Verification items for the finished model (mm, model axes). A direction names the side the tool comes from. Coordinates: 2 decimals unless noted, no trailing zeros. Order: outer loops, then holes, each group sorted by start corner. A loop starts at its lowest first (then second) coordinate and runs counter-clockwise, first axis right, second up. Notation, with made-up numbers: M 2,-2 L 43,-2 A18 cw 43,21 Z; hole C 68.25,-11.75 d6. An arc over 180 degrees is marked long. Return JSON: item names as keys, results as strings. Group by question number.
1. Section check D-D, the plane y = 8.5. Record the cut outline in (x, z).
2. Section check A-A, the plane z = 70. Record the cut outline in (x, y).
3. Material ranges on line 1 along X through (y, z) = (36, 40.5); line 2 along Z through (x, y) = (41.5, 30); line 3 along Y through (x, z) = (-38, 90), recorded low to high.
4. Gauge pin test, flat ends, axial feed: pin 1 (10 mm diameter, centred on x = -9.5, y = 20, fed in from -Z); pin 2 (22 mm diameter, centred on y = 31, z = 50.5, fed in from +X); pin 3 (7 mm diameter, centred on y = 37, z = 79.5, fed in from -X). Record the tip position at first contact, or that the pin passes through.
5. Section check B-B, the plane x = 20. Record the cut outline in (y, z).
6. Set-up check for faces 1 (the cylindrical face through (40.56, 20.917, -6.377)), 2 (the flat face through (-14, 25.981, 15)), 3 (the flat face through (-40, 33, 69)): record each of +Z, -Z, +X, -X, +Y, -Y from which the full face is reachable in a straight line by a thin tool's end or side.
7. Section check C-C, the plane z = 50. Record the cut outline in (x, y), plus the area to 3 significant figures.
8. Mould release check, pull along X, two halves, no side actions. Record for faces 4 (the cylindrical face through (-29.191, -19.984, 69.44)), 5 (the cylindrical face through (56.315, 36.292, -7.465)), 6 (the flat face through (80, 19, -11)), 7 (the flat face through (41, 34, 10)): +X half, -X half, draft (parallel to the pull), parting line (faces both ways), or undercut.
```python
from build123d import *

# Parameters (mm, degrees)
BOSS_EXTRUDE1_DEPTH = 80
SKETCH2_R           = 5
CUT_EXTRUDE1_DEPTH  = 10
FILLET2_R           = 5
FILLET3_R           = 10
BOSS_EXTRUDE2_START = 25.98076
BOSS_EXTRUDE2_DEPTH = 16.932117
FILLET4_R           = 20
FILLET5_R           = 25
SKETCH6_W           = 5
SKETCH6_H           = 16.932118475
BOSS_EXTRUDE4_DEPTH = 80
SKETCH7_R           = 5
CUT_EXTRUDE2_DEPTH  = 40


with BuildPart() as part:
    # Sketch1 → Boss-Extrude1 (new body)
    with BuildSketch(Plane(origin=(0, 0, 0), x_dir=(0, 0, -1), z_dir=(1, 0, 0))):
        with BuildLine():
            Line((-10, 22.912878475), (-10, 42.912878475))
            Line((-10, 42.912878475), (-5, 42.912878475))
            Line((-5, 42.912878475), (-5, 19.364916731))
            ThreePointArc((-5, 19.364916731), (0, -20), (5, 19.364916731))
            Line((5, 19.364916731), (5, 42.912878475))
            Line((5, 42.912878475), (10, 42.912878475))
            Line((10, 42.912878475), (10, 22.912878475))
            ThreePointArc((10, 22.912878475), (0, -25), (-10, 22.912878475))
        make_face()
    extrude(amount=BOSS_EXTRUDE1_DEPTH)

    # Sketch2 → Cut-Extrude1 (cut, symmetric)
    with BuildSketch(Plane.XY):
        with Locations((20, 32.912878475)):
            Circle(SKETCH2_R)
        with Locations((60, 32.912878475)):
            Circle(SKETCH2_R)
    extrude(amount=CUT_EXTRUDE1_DEPTH, both=True, mode=Mode.SUBTRACT)

    # Fillet2
    fillet2_edges = [part.edges().sort_by_distance(p)[0] for p in [
        (40, 22.912878475, -10),
        (40, 22.912878475, 10),
    ]]
    fillet(fillet2_edges, radius=FILLET2_R)

    # Fillet3
    fillet3_edges = [part.edges().sort_by_distance(p)[0] for p in [
        (40, 19.364916731, 5),
        (40, 19.364916731, -5),
    ]]
    fillet(fillet3_edges, radius=FILLET3_R)

    # Sketch3 → Boss-Extrude2 (add)
    with BuildSketch(Plane(origin=(0, 0, 0), x_dir=(1, 0, 0), z_dir=(0, 1, 0)).offset(BOSS_EXTRUDE2_START)):
        Polygon((0, -10), (-20, -10), (-20, -30), (-25, -30), (-25, -5), (0, -5), align=None)
    extrude(amount=BOSS_EXTRUDE2_DEPTH)

    # Fillet4
    fillet4_edges = [part.edges().sort_by_distance(p)[0] for p in [
        (-20, 34.4468185, 10),
    ]]
    fillet(fillet4_edges, radius=FILLET4_R - 0.0001)  # a hair under: the kernel refuses the full size

    # Fillet5
    fillet5_edges = [part.edges().sort_by_distance(p)[0] for p in [
        (-25, 34.4468185, 5),
    ]]
    fillet(fillet5_edges, radius=FILLET5_R - 0.0001)  # a hair under: the kernel refuses the full size

    # Sketch6 → Boss-Extrude4 (add)
    with BuildSketch(Plane.XY.offset(30)):
        with BuildLine():
            Line((-20, 25.98076), (-25, 25.98076))
            Line((-25, 25.98076), (-25, 19.364916731))
            ThreePointArc((-25, 19.364916731), (-30, -20), (-35, 19.364916731))
            Line((-35, 19.364916731), (-35, 42.912878475))
            Line((-35, 42.912878475), (-40, 42.912878475))
            Line((-40, 42.912878475), (-40, 22.912878475))
            ThreePointArc((-40, 22.912878475), (-30, -25), (-20, 22.912878475))
            Line((-20, 22.912878475), (-20, 25.98076))
        make_face()
        with Locations((-22.5, 34.446819238)):
            Rectangle(SKETCH6_W, SKETCH6_H)
    extrude(amount=BOSS_EXTRUDE4_DEPTH)

    # Sketch7 → Cut-Extrude2 (cut)
    with BuildSketch(Plane(origin=(0, 0, 0), x_dir=(0, 0, -1), z_dir=(1, 0, 0))):
        with Locations((-90, 32.912878475)):
            Circle(SKETCH7_R)
        with Locations((-50, 32.912878475)):
            Circle(SKETCH7_R)
    extrude(amount=-CUT_EXTRUDE2_DEPTH, mode=Mode.SUBTRACT)


solid = part.part
```
Answers follow:
{
 "1": {"outline": "M -53.51,30 L -48.1,30 L -48.1,110 L -53.51,110 Z; M -11.9,30 L -6.49,30 L -6.49,110 L -11.9,110 Z; M 0,-23.51 L 80,-23.51 L 80,-18.1 L 0,-18.1 Z; M 0,18.1 L 80,18.1 L 80,23.51 L 0,23.51 Z"},
 "2": {"outline": "M -40,22.91 A25 ccw long -20,22.91 L -20,42.91 L -25,42.91 L -25,19.36 A20 cw long -35,19.36 L -35,42.91 L -40,42.91 Z"},
 "3": {"line 1": "-40 to -35, -25 to -20", "line 2": "-10 to -5, 5 to 10", "line 3": "-23.69 to -18.33, 18.33 to 27.91, 37.91 to 42.91"},
 "4": {"pin 1": "z = 30", "pin 2": "x = -15", "pin 3": "x = -40"},
 "5": {"outline": "M 17.32,-10 A20 cw long 17.32,10 A10 ccw 25.98,5 L 27.91,5 L 27.91,10 L 25.98,10 A5 cw 21.65,12.5 A25 ccw long 21.65,-12.5 A5 cw 25.98,-10 L 27.91,-10 L 27.91,-5 L 25.98,-5 A10 ccw Z; M 37.91,-10 L 42.91,-10 L 42.91,-5 L 37.91,-5 Z; M 37.91,5 L 42.91,5 L 42.91,10 L 37.91,10 Z"},
 "6": {"face 1": "+X, -X", "face 2": "-Z, -X, -Y", "face 3": "+Z, -Z, -X, +Y"},
 "7": {"outline": "M -40,22.91 A25 ccw long -20,22.91 L -20,27.91 L -25,27.91 L -25,19.36 A20 cw long -35,19.36 L -35,27.91 L -40,27.91 Z; M -40,37.91 L -35,37.91 L -35,42.91 L -40,42.91 Z; M -25,37.91 L -20,37.91 L -20,42.91 L -25,42.91 Z", "area": "748 mm^2"},
 "8": {"face 4": "undercut", "face 5": "undercut", "face 6": "+X half", "face 7": "draft"}
}
